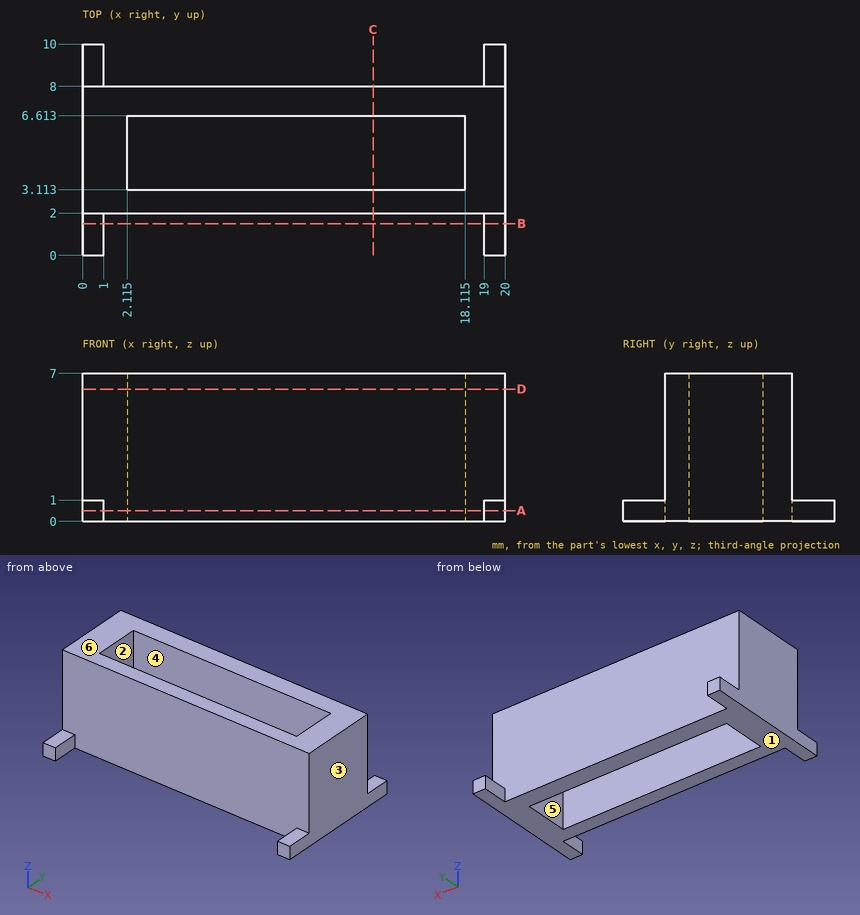
For this review, use the dimensioned drawing (mm, ordinates from the lowest corner) and the shaded views. A direction names the side the tool comes from. Coordinates: 2 decimals unless noted, no trailing zeros. Loops run counter-clockwise (first coordinate to the right, second up) from the corner with the lowest first, then second, coordinate; pieces in that order, holes last. Notation, with made-up numbers: (23, 76.5) -> (33, 76.5) arc R15 ccw to (33, 82.5) -> close; hole circle Ø1 at (34.25, -1). An arc over 180 degrees is marked (long way). Use a Markdown table: item, result. Add a question column.
Item 1: Machinability: for the marked faces 5 and 6, which of the approach directions +Z, -Z, +X, -X, +Y, -Y give a long, thin tool a straight path to every point of the face, cutting with its end or side? Answer none if there is none.
Item 2: We need section A-A, the plane z = 0.5. Write out the cut boundary in (x, y) (1 decimal).
Item 3: The part is to be moulded in two halves that separate along X. For the marked faces 1, 2, 3 and 4, say which applies: +X half, -X half, draft (parallel to the pull), parting line (faces both ways), or undercut.
Item 4: We need section C-C, the plane x = 13.75. Write out the cut boundary in (y, z).
Item 5: Clearance check with flat-ended pins moving along their axes: P1, Ø1.1, axis at x = 0.5, y = 0.5, coming from the +Z side; P2, Ø3.5, axis at x = 10.5, z = 3.5, coming from the -Y side; P3, Ø1, axis at x = 11, y = 6.5, coming from the +Z side; P4, Ø2, axis at x = 9, z = 2, coming from the +Y side. State where each tip first meets the part, or that it passes through.
Item 6: Wall thickness on L1, parallel to Y at x = 17.25, z = 2.25; L2, parallel to X at y = 3.25, z = 2.25 (1 decimal); L3, parallel to Y at x = 1.75, z = 5.5: over which ranges is each line inside the solid? List them lowest first. Write a range as from..to.
Item 7: We need section B-B, the plane y = 1.5. Write out the cut boundary in (x, z).
Item 8: We need section D-D, the plane z = 6.25. Write out the cut boundary in (x, y) (1 decimal).
Numbers:
| question | item | result |
|---|---|---|
| 1 | face 5 | +Z, -Z |
| 1 | face 6 | +Z, +X, -X, +Y, -Y |
| 2 | outline | (0, 0) -> (1, 0) -> (1, 2) -> (19, 2) -> (19, 0) -> (20, 0) -> (20, 10) -> (19, 10) -> (19, 8) -> (1, 8) -> (1, 10) -> (0, 10) -> close; hole (2.1, 3.1) -> (18.1, 3.1) -> (18.1, 6.6) -> (2.1, 6.6) -> close |
| 3 | face 1 | draft |
| 3 | face 2 | undercut |
| 3 | face 3 | +X half |
| 3 | face 4 | undercut |
| 4 | outline | (2, 0) -> (3.11, 0) -> (3.11, 7) -> (2, 7) -> close; (6.61, 0) -> (8, 0) -> (8, 7) -> (6.61, 7) -> close |
| 5 | P1 | stops at z = 1 |
| 5 | P2 | stops at y = 2 |
| 5 | P3 | stops at z = 7 |
| 5 | P4 | stops at y = 8 |
| 6 | L1 | y = 2..3.11, 6.61..8 |
| 6 | L2 | x = 0..2.1, 18.1..20 |
| 6 | L3 | y = 2..8 |
| 7 | outline | (0, 0) -> (1, 0) -> (1, 1) -> (0, 1) -> close; (19, 0) -> (20, 0) -> (20, 1) -> (19, 1) -> close |
| 8 | outline | (0, 2) -> (20, 2) -> (20, 8) -> (0, 8) -> close; hole (2.1, 3.1) -> (18.1, 3.1) -> (18.1, 6.6) -> (2.1, 6.6) -> close |
